Here's how the part is built. I have some questions about the finished solid (model axes, mm). A direction names the side the tool comes from. Coordinates: 2 decimals unless noted, no trailing zeros. Loops run counter-clockwise (first coordinate to the right, second up) from the corner with the lowest first, then second, coordinate; pieces in that order, holes last. Notation, with made-up numbers: M -17,35.5 L 34,35.5 A30 cw 34,61.5 Z; hole C -38.75,-17 d1. An arc over 180 degrees is marked long. Use one line per item in the form item = value. Start each with the question number.
(1) On a 3-axis mill with a long thin cutter (end or side, diameter ignored), from which of +Z, -Z, +X, -X, +Y, -Y can I reach the whole of each face in a straight line? I mean faces 1 (the flat face through (7, 2, 12)), 2 (the flat face through (-490, 8, 1)). Say none if no direction works.
(2) Please list where these lines run through material, in increasing order: L1, parallel to Z at x = 225.5, y = 26; L2, parallel to Z at x = -362, y = 4.
(3) Will these pins go through, and if not, where does the flat tip stop? P1, Ø5, axis at x = 108.5, z = 13, coming from the +Y side; P2, Ø1, axis at x = -245.5, z = 0.5, coming from the +Y side; P3, Ø2, axis at y = 37.5, z = 1.5, coming from the -X side; P4, Ø1.5, axis at y = 20.5, z = 3, coming from the -X side.
(4) Imagine slicing it at A-A, the plane y = 35.5. Please give me the cut outline in (x, z), and give its area (3 significant figures).
(5) Imagine slicing it at C-C, the plane z = 17. Please give me the cut outline in (x, y), and give its area (3 significant figures).
(6) Imagine slicing it at B-B, the plane x = 292.5. Please give me the cut outline in (y, z).
Autodesk Inventor part; units mm, degrees
ref_plane "YZ Plane" through (0, 0, 0) normal (1, 0, 0) x (0, 1, 0)
ref_plane "XZ Plane" through (0, 0, 0) normal (0, 1, 0) x (-1, 0, 0)
ref_plane "XY Plane" through (0, 0, 0) normal (0, 0, 1) x (1, 0, 0)
sketch "Sketch1" plane through (0, 0, 0) normal (0, 0, 1) x (1, 0, 0)
  line L0 (-490, 59) -> (490, 59)
  line L1 (490, 59) -> (490, 0)
  line L2 (490, 0) -> (-490, 0)
  line L3 (-490, 0) -> (-490, 59)
  point P0 (0, 0)
  point P1 (0, 0)
  dimension "d0" = 980
  dimension "d1" = 59
extrude "Plate1" add sketch "Sketch1" along normal blind 2
sketch "Sketch2" plane through (490, 2, 0) normal (0, -1, 0) x (1, 0, 0)
  line L0 (-980, 0) -> (0, 0)
  line L1 (0, 0) -> (0, 20)
  line L2 (0, 20) -> (-980, 20)
  line L3 (-980, 20) -> (-980, 0)
edge flange "Flange1" height 20 angle 90 thickness 2 bend radius 2.75 thickness toward (0, -1, 0) relief round relief width 2 relief depth 1 edges at (0, 0, 2) wall of the first edge with corners at (-490, 2, 0) (490, 2, 0) (490, 2, 20) (-490, 2, 20)
bend "Bend1"
corner "Corner1"
sketch "Sketch5" plane through (0, 0, 0) normal (0, 0, -1) x (-1, 0, 0)
  line L0 (490, 59) -> (-490, 59)
  line L1 (490, 0) -> (-490, 0)
  circle A0 centre (0, 59) radius 35
  line L2 (243.95, 59) -> (246.05, 59)
  line L3 (246.05, 59) -> (246.05, 27)
  line L4 (246.05, 27) -> (243.95, 27)
  line L5 (243.95, 27) -> (243.95, 59)
  line L6 (-243.95, 59) -> (-246.05, 59)
  line L7 (-246.05, 59) -> (-246.05, 27)
  line L8 (-246.05, 27) -> (-243.95, 27)
  line L9 (-243.95, 27) -> (-243.95, 59)
  line L10 (0, 59) -> (0, 0) construction
  circle A1 centre (-490, 59) radius 35
  circle A2 centre (490, 59) radius 35
  point P0 (0, 0)
  point P1 (245, 27)
  point P2 (-245, 27)
  point P3 (246.05, 59)
  point P4 (-35, 59)
  point P5 (35, 59)
  point P6 (-246.05, 59)
  dimension "d45" = 70
  dimension "d48" = 2.1
  dimension "d49" = 490
  dimension "d51" = 27
  dimension "d52" = 32
extrude "Extrusion1" cut sketch "Sketch5" against normal through all contours L3 L4 L5 L0 | L9 L8 L7 L0 | A2
sketch "Sketch9" plane through (0, 0, 2) normal (0, 0, 1) x (1, 0, 0)
  line L0 (485.6141, 29.596) -> (485.6141, 17.596) construction
  line L1 (485.6141, 17.596) -> (285.6141, 17.596) construction
  line L2 (285.6141, 17.596) -> (285.6141, 29.596) construction
  line L3 (285.6141, 29.596) -> (485.6141, 29.596) construction
  line L4 (-490, 59) -> (490, 59)
  point P0 (0, 0)
  point P1 (1.05, 68)
  point P2 (490, 59)
  dimension "d40" = 200
  dimension "d41" = 12
mark "Mark2"
equation "\"d2\" = Thickness"
equation "\"d3\" = BendReliefWidth"
equation "\"d4\" = BendReliefDepth"
equation "\"d5\" = MinimumRemnant"
equation "\"d6\" = TransitionRadius"
equation "\"d9\" = BendRadius"
equation "\"d10\" = CornerReliefSize"
equation "\"d11\" = GapSize"
equation "\"d12\" = JacobiRadiusSize"
equation "\"BendReliefWidth\" = Thickness"
equation "\"BendReliefDepth\" = 0.5 * Thickness"
equation "\"CornerReliefSize\" = 4 * Thickness"
equation "\"MinimumRemnant\" = 2 * Thickness"
equation "\"TransitionRadius\" = BendRadius"
equation "\"JacobiRadiusSize\" = BendRadius"
equation "\"GapSize\" = Thickness"
properties part number "MSC 323 STRINGER BOARD  #" material "Stainless Steel"
Answer:
q1.face_1 = +Z, +X, -X, +Y
q1.face_2 = +Z, -Z, -X, +Y, -Y
q2.L1 = 0 to 2
q2.L2 = 0.06 to 2.1
q3.P1 = 2
q3.P2 = 27
q3.P3 = -463.19
q3.P4 = through
q4.outline = M -464.06,0 L -246.05,0 L -246.05,2 L -464.06,2 Z; M -243.95,0 L 243.95,0 L 243.95,2 L -243.95,2 Z; M 246.05,0 L 490,0 L 490,2 L 246.05,2 Z
q4.area = 1,900 mm²
q5.outline = M -490,0 L 490,0 L 490,2 L -490,2 Z
q5.area = 1,960 mm²
q6.outline = M 0,4.75 A4.75 ccw 4.75,0 L 59,0 L 59,2 L 4.75,2 A2.75 cw 2,4.75 L 2,20 L 0,20 Z
